Source: three-view drawing plus pictorial views. Frame: mm from the lowest corner of the part. A direction names the side the tool comes from. Give positions to 0.01 mm unless a question says otherwise; leave off trailing zeros. Order: outer loops, then holes, each group sorted by start corner. A loop starts at its lowest first (then second) coordinate and runs counter-clockwise, first axis right, second up. Notation, with made-up numbers: (33.5, -39.5) - (90.5, -39.5) arc R22 cw to (90.5, -12.5) - close; hole circle Ø3 at (66.5, -28.75). An arc over 180 degrees is marked (long way). Use CSV: the item, a comma, the result in double quotes.
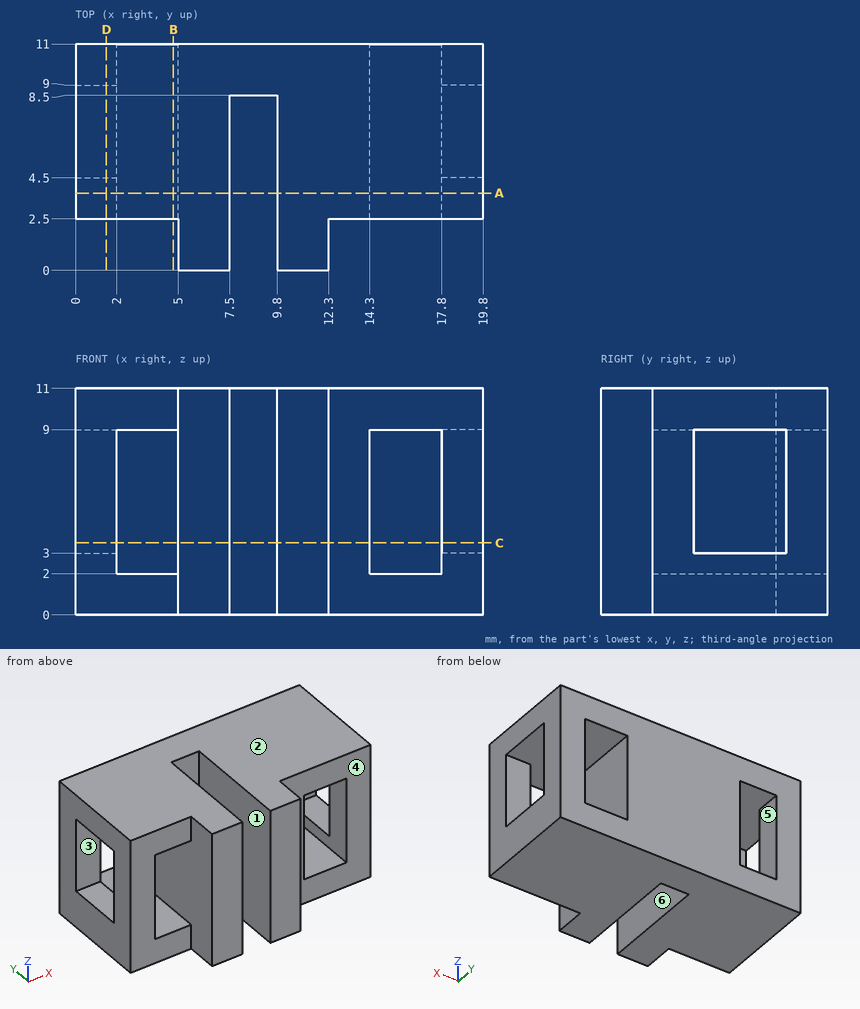
Item 1: Section C-C on z = 3.5. Return the cut outline in (x, y).
Filled in:
outline,"(0, 2.5) - (2, 2.5) - (2, 4.5) - (0, 4.5) - close; (0, 9) - (2, 9) - (2, 11) - (0, 11) - close; (5, 0) - (7.5, 0) - (7.5, 8.5) - (9.8, 8.5) - (9.8, 0) - (12.3, 0) - (12.3, 2.5) - (14.3, 2.5) - (14.3, 11) - (5, 11) - close; (17.8, 2.5) - (19.8, 2.5) - (19.8, 4.5) - (17.8, 4.5) - close; (17.8, 9) - (19.8, 9) - (19.8, 11) - (17.8, 11) - close"
Item 2: Material intervals for line 1 (X direction, y = 9.5, z = 3.5); line 2 (Y direction, x = 1.5, z = 4.25); line 3 (X direction, y = 2, z = 2), sorted ascending. Write a range as from..to.
Filled in:
line 1,"x = 0..2, 5..14.3, 17.8..19.8"
line 2,"y = 2.5..4.5, 9..11"
line 3,"x = 5..7.5, 9.8..12.3"
Item 3: Set-up query: the marked faces 4, 5 and 6. Return all of +Z, -Z, +X, -X, +Y, -Y with unobstructed straight access to the full face (end or side cutting, diameter ignored); none if empty.
Filled in:
face 4,"+Z, -Z, +X, -Y"
face 5,"+Y, -Y"
face 6,"+Z, -Z, -Y"
Item 4: Mould query, pull axis Z, two halves, no side actions, for the marked faces 1, 2 and 3. Classes: released by +Z, released by -Z, zero draft, split by the parting line, or undercut.
Filled in:
face 1,"zero draft"
face 2,"released by +Z"
face 3,"undercut"
Item 5: Section D-D on x = 1.5. Return the cut outline in (y, z).
Filled in:
outline,"(2.5, 0) - (11, 0) - (11, 11) - (2.5, 11) - close; hole (4.5, 3) - (9, 3) - (9, 9) - (4.5, 9) - close"
Item 6: First-contact query: pin 1 (2.5 mm diameter, centred on x = 9, z = 4, fed in from -Y); pin 2 (1 mm diameter, centred on x = 18.5, z = 7, fed in from -Y). Flat tips, straight axial feed; report the tip coordinate or a pass-through.
Filled in:
pin 1,"stops at y = 0"
pin 2,"stops at y = 2.5"
Item 7: Section B-B on x = 4.75. Return the cut outline in (y, z), then the cut area to 3 significant figures.
Filled in:
outline,"(2.5, 0) - (11, 0) - (11, 2) - (2.5, 2) - close; (2.5, 9) - (11, 9) - (11, 11) - (2.5, 11) - close"
area,"34.0 mm2"
Item 8: Section A-A on y = 3.75. Return the cut outline in (x, z), then the cut area to 3 significant figures.
Filled in:
outline,"(0, 0) - (7.5, 0) - (7.5, 11) - (0, 11) - close; (9.8, 0) - (19.8, 0) - (19.8, 11) - (9.8, 11) - close; hole (2, 2) - (5, 2) - (5, 9) - (2, 9) - close; hole (14.3, 2) - (17.8, 2) - (17.8, 9) - (14.3, 9) - close"
area,"147 mm2"
